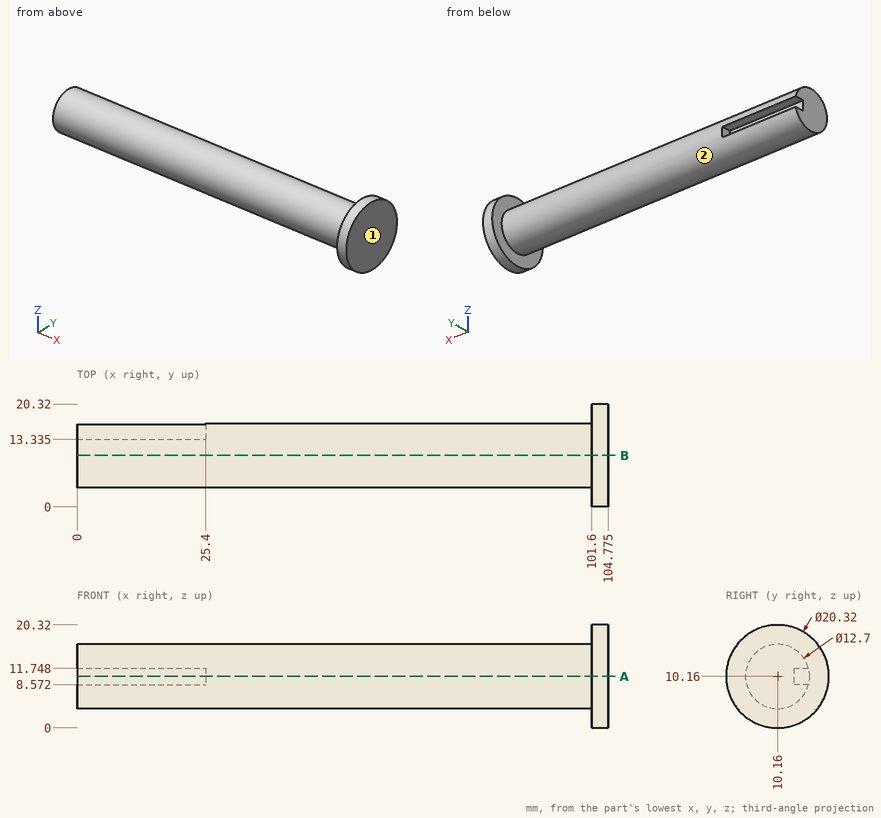
The figure shows three views and two pictorial views of one solid part (mm, origin at its lowest corner). Answer the questions. A direction names the side the tool comes from. Give positions to 0.01 mm unless a question says otherwise; leave off trailing zeros. Loops run counter-clockwise (first coordinate to the right, second up) from the corner with the lowest first, then second, coordinate; pieces in that order, holes last. Notation, with made-up numbers: (56, 20) - (62, 20) arc R20 cw to (62, 59) - close; hole circle Ø3 at (48.25, 30). An arc over 180 degrees is marked (long way). Answer in a Markdown table with one row per item.
(1) A tool of negligible diameter and unlimited length cuts with its end or side. For the marked faces 1 and 2, from which of +Z, -Z, +X, -X, +Y, -Y can it reach the whole face along a straight path? Write none if from no direction.
Results list:
| item | result |
|---|---|
| face 1 | +Z, -Z, +X, +Y, -Y |
| face 2 | -X |
(2) Consider L1, parallel to X at y = 12, z = 3.75 (1 decimal); L2, parallel to Y at x = 23, z = 12.5; L3, parallel to Y at x = 79, z = 15.25 (1 decimal). Determine where each line is inside the solid, lowest interval first. Write a range as [from, to].
Results list:
| item | result |
|---|---|
| L1 | x = [101.6, 104.8] |
| L2 | y = [4.26, 16.06] |
| L3 | y = [6.4, 14] |
(3) Flat-ended cylindrical pins translate along their axes: pin 1 Ø2 at (x, y) = (91.5, 2.5) entering from +Z; pin 2 Ø1.5 at (x, y) = (16, 14) entering from +Z; pin 3 Ø1 at (x, z) = (32, 8) entering from -Y; pin 4 Ø3 at (y, z) = (2.5, 18.5) entering from -X. Find the tip coordinate at first contact, or state that the pin passes through.
Results list:
| item | result |
|---|---|
| pin 1 | passes through |
| pin 2 | stops at z = 15.71 |
| pin 3 | stops at y = 4.03 |
| pin 4 | stops at x = 101.6 |
(4) Section B-B (y = 10.16) is taken. Give the vertices of the cut face in (x, z) (1 decimal).
Results list:
| item | result |
|---|---|
| outline | (0, 3.8) - (101.6, 3.8) - (101.6, 0) - (104.8, 0) - (104.8, 20.3) - (101.6, 20.3) - (101.6, 16.5) - (0, 16.5) - close |
(5) Section A-A (z = 10.16) is taken. Give the vertices of the cut face in (x, y) (1 decimal).
Results list:
| item | result |
|---|---|
| outline | (0, 3.8) - (101.6, 3.8) - (101.6, 0) - (104.8, 0) - (104.8, 20.3) - (101.6, 20.3) - (101.6, 16.5) - (25.4, 16.5) - (25.4, 13.3) - (0, 13.3) - close |
